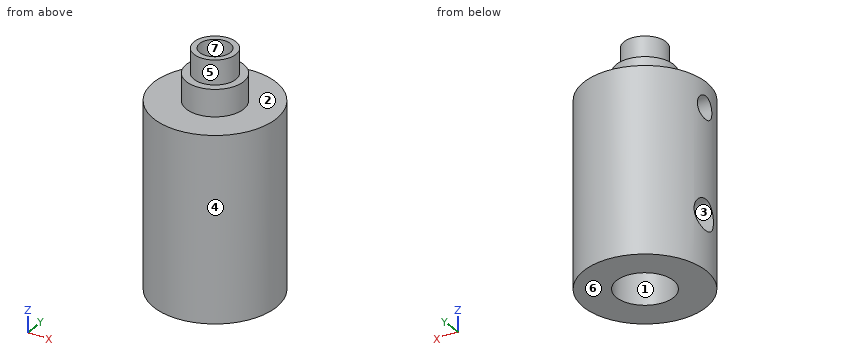
```python
from build123d import *

# Parameters (mm, degrees)
F0_R      = 5.5
F0_R_2    = 4
F1_DEPTH  = 6.36
F2_R      = 16
F2_R_2    = 5.5
F2_R_3    = 4
F3_DEPTH  = 55
F4_R      = 36.2915386418
F4_R_2    = 16
F4_R_3    = 7.5
F5_DEPTH  = 7
F6_R      = 3
F7_DEPTH  = 25
F8_R      = 7.45
F8_R_2    = 4
F9_DEPTH  = 24
F10_R     = 4
F11_DEPTH = 25


with BuildPart() as f1:
    # F0 (on Top) → F1 (new body)
    with BuildSketch(Plane.XY):
        Circle(F0_R)
        Circle(F0_R_2, mode=Mode.SUBTRACT)
    extrude(amount=F1_DEPTH)

    # F2 (on face) → F3 (join)
    with BuildSketch(Plane(origin=(0, 0, 0), x_dir=(1, 0, 0), z_dir=(0, 0, -1))):
        Circle(F2_R)
        Circle(F2_R_2, mode=Mode.SUBTRACT)
        Circle(F2_R_2)
        Circle(F2_R_3, mode=Mode.SUBTRACT)
    extrude(amount=F3_DEPTH)

    # F4 (on face) → F5 (cut)
    with BuildSketch(Plane.XY):
        Circle(F4_R)
        Circle(F4_R_2, mode=Mode.SUBTRACT)
        Circle(F4_R_2)
        Circle(F4_R_3, mode=Mode.SUBTRACT)
    extrude(amount=-F5_DEPTH, mode=Mode.SUBTRACT)

    # F6 (on Right) → F7 (cut)
    with BuildSketch(Plane.YZ):
        with Locations((0, -13.64)):
            Circle(F6_R)
    extrude(amount=-F7_DEPTH, mode=Mode.SUBTRACT)

    # F8 (on face) → F9 (cut)
    with BuildSketch(Plane(origin=(0, 0, -55), x_dir=(1, 0, 0), z_dir=(0, 0, -1))):
        Circle(F8_R)
        Circle(F8_R_2, mode=Mode.SUBTRACT)
    extrude(amount=-F9_DEPTH, mode=Mode.SUBTRACT)

    # F10 (on Right) → F11 (cut)
    with BuildSketch(Plane.YZ):
        with Locations((0, -40.9)):
            Circle(F10_R)
    extrude(amount=-F11_DEPTH, mode=Mode.SUBTRACT)


solid = f1.part
```
Design review of the part built by this model. Coordinates are the model's own, in mm. Face numbers are marked on the shaded views. A direction names the side the tool comes from. Give positions to 0.01 mm unless a question says otherwise; leave off trailing zeros. Write each loop counter-clockwise with the first axis right and the second up, starting at its lowest first coordinate (ties: lowest second). Pieces come first, ordered by that corner, then holes. Notation, with made-up numbers: (-27.5, 5) - (-5.5, 5) arc R25 ccw to (-5.5, 21) - close; hole circle Ø7 at (-17, 30). An arc over 180 degrees is marked (long way). Return JSON: item names as keys, results as strings. Group by question number.
(1) We need section C-C, the plane z = -5. Give the boundary of the cut face in (x, y), then the cut area to 3 significant figures.
(2) Mouldability with a two-part tool opening along X and no side actions: class the marked faces 5, 6 and 7 as +X half, -X half, draft (parallel to the pull), parting line (faces both ways), or undercut.
(3) We need section D-D, the plane z = -28.5. Give the boundary of the cut face in (x, y), then the cut area to 3 significant figures.
(4) Insertion check: pin 1 (6 mm diameter, centred on y = -7.5, z = -25.5, fed in from +X); pin 2 (2 mm diameter, centred on x = -2.5, y = 5.5, fed in from -Z); pin 3 (12 mm diameter, centred on x = 11.5, z = -35.5, fed in from +Y) (3 decimals). Each pin has a flat end and moves straight along its axis. Give the tip position at first contact, or say it passes through.
(5) We need section B-B, the plane x = 0. Give the boundary of the cut face in (y, z), then the cut area to 3 significant figures.
(6) We need section A-A, the plane y = 0. Give the boundary of the cut face in (x, z).
(7) Machinability: for the marked faces 1, 2, 3 and 4, which of the approach directions +Z, -Z, +X, -X, +Y, -Y give a long, thin tool a straight path to every point of the face, cutting with its end or side? Answer none if there is none.
(8) To check wall thickness, follow probe 1 along Y at (x, z) = (0, -42); probe 2 along X at (y, z) = (0, -9). State the ranges of each line that lie inside material, in increasing order.
Reported:
{
 "1": {"outline": "circle Ø15 at (0, 0); hole circle Ø8 at (0, 0)", "area": "126 mm2"},
 "2": {"face 5": "parting line", "face 6": "draft", "face 7": "undercut"},
 "3": {"outline": "circle Ø32 at (0, 0); hole circle Ø8 at (0, 0)", "area": "754 mm2"},
 "4": {"pin 1": "stops at x = 15.35", "pin 2": "stops at z = -31", "pin 3": "stops at y = 15.025"},
 "5": {"outline": "(-16, -55) - (-7.45, -55) - (-7.45, -31) - (-4, -31) - (-4, 6.36) - (-5.5, 6.36) - (-5.5, 0) - (-7.5, 0) - (-7.5, -7) - (-16, -7) - close; (4, -31) - (7.45, -31) - (7.45, -55) - (16, -55) - (16, -7) - (7.5, -7) - (7.5, 0) - (5.5, 0) - (5.5, 6.36) - (4, 6.36) - close", "area": "1,050 mm2"},
 "6": {"outline": "(-16, -55) - (-7.45, -55) - (-7.45, -44.9) - (-16, -44.9) - close; (-16, -36.9) - (-7.45, -36.9) - (-7.45, -31) - (-4, -31) - (-4, -16.64) - (-16, -16.64) - close; (-16, -10.64) - (-4, -10.64) - (-4, 6.36) - (-5.5, 6.36) - (-5.5, 0) - (-7.5, 0) - (-7.5, -7) - (-16, -7) - close; (4, -31) - (7.45, -31) - (7.45, -55) - (16, -55) - (16, -7) - (7.5, -7) - (7.5, 0) - (5.5, 0) - (5.5, 6.36) - (4, 6.36) - close"},
 "7": {"face 1": "-Z", "face 2": "+Z", "face 3": "-X", "face 4": "+Z, -Z"},
 "8": {"probe 1": "y = -16 to -7.45, 7.45 to 16", "probe 2": "x = -16 to -4, 4 to 16"}
}
